Can you work these out from the model? Positions are in its coordinate system, mm. Face numbers are marked on the shaded views. A direction names the side the tool comes from. Give positions to 0.01 mm unless a question says otherwise; leave off trailing zeros. Write each loop counter-clockwise with the first axis right and the second up, starting at its lowest first coordinate (ties: lowest second). Pieces come first, ordered by that corner, then holes.
1. I'm going to push flat-ended pins straight in: pin 1 (2.5 mm diameter, centred on x = 0, z = 10, fed in from -Y); pin 2 (5 mm diameter, centred on x = -50, z = 10, fed in from -Y); pin 3 (2 mm diameter, centred on x = -53.5, y = -2.5, fed in from +Z); pin 4 (4 mm diameter, centred on x = -27.5, z = 8, fed in from -Y). Where does each tip first touch, or does it pass through?
2. Suppose I cut it at A-A (x = -50). Please give me the cut outline in (y, z), and give its area (3 significant figures).
3. If I drill on probe 1 along Z at (x, y) = (-50, -2.4); probe 2 along X at (y, z) = (-1.5, 9.75); probe 3 along Z at (x, y) = (-11, -5.5), over which ranges is the centre line in solid material (lowest first)?
4. On a 3-axis mill with a long thin cutter (end or side, diameter ignored), from which of +Z, -Z, +X, -X, +Y, -Y can I reach the whole of each face in a straight line? I mean the marked faces 5 and 6. Say none if no direction works.
5. Suppose I cut it at B-B (y = -0.5). Please give me the cut outline in (x, z).
6. Suppose I cut it at C-C (z = 10). Please give me the cut outline in (x, y), and give its area (3 significant figures).
7. Suppose I cut it at D-D (x = -41). Please give me the cut outline in (y, z).
8. Thinking about a two-plate mould opening in X: for the marked faces 1, 2, 3 and 4, which applies, pulls with the +X half, pulls with the -X half, needs draft (parallel to the pull), parting line crosses it, or undercut?
```python
from build123d import *

# Parameters (mm, degrees)
F0_R         = 1.5
F1_DEPTH     = 8
F2_T1_DEPTH  = 17.5
F2_T3_DEPTH  = 70
F2_T5_DEPTH  = 7
F2_T7_DEPTH  = 10
F2_T9_DEPTH  = 16
F2_T11_DEPTH = 44
F2_T13_DEPTH = 16
F2_T15_DEPTH = 7
F2_T25_DEPTH = 12
F2_T29_DEPTH = 15
F2_T36_DEPTH = 15
F2_T40_DEPTH = 49
F2_T47_DEPTH = 49
F2_T51_DEPTH = 15
F2_T58_DEPTH = 15
F2_T62_DEPTH = 12


# Not quite as in the source:
# - a fillet or chamfer that OpenCascade refuses, or shapes differently, is made with other operations: its cross-section is extruded or revolved along the edge and cut away or added


with BuildPart() as f1:
    # F0 (on Front) → F1 (new body)
    with BuildSketch(Plane.XZ):
        Polygon((-55, 7.5), (-55, 0), (5, 0), (5, 7.5), (3, 7.5), (3, 12.5), (-3, 12.5), (-3, 7.5), (-47, 7.5), (-47, 12.5), (-53, 12.5), (-53, 7.5), align=None)
        with Locations((-50, 10)):
            Circle(F0_R, mode=Mode.SUBTRACT)
        with Locations((0, 10)):
            Circle(F0_R, mode=Mode.SUBTRACT)
    extrude(amount=F1_DEPTH)

    # F2: fillet of radius 2 on 14 edges, made by hand

    # F2_s2 → F2_t1 (cut)
    with BuildSketch(Plane.XY.offset(-5)):
        with BuildLine():
            ThreePointArc((-55, -6), (-54.4142135624, -7.4142135624), (-53, -8))
            Line((-53, -8), (-55, -8))
            Line((-55, -8), (-55, -6))
        make_face()
        with BuildLine():
            ThreePointArc((5, -6), (4.4142135624, -7.4142135624), (3, -8))
            Line((3, -8), (5, -8))
            Line((5, -8), (5, -6))
        make_face()
    extrude(amount=F2_T1_DEPTH, mode=Mode.SUBTRACT)

    # F2_s4 → F2_t3 (cut)
    with BuildSketch(Plane.YZ.offset(-60)):
        with BuildLine():
            ThreePointArc((-6, 0), (-7.4142135624, 0.5857864376), (-8, 2))
            Line((-8, 2), (-8, 0))
            Line((-8, 0), (-6, 0))
        make_face()
    extrude(amount=F2_T3_DEPTH, mode=Mode.SUBTRACT)

    # F2_s6 → F2_t5 (cut)
    with BuildSketch(Plane.YZ.offset(3)):
        with BuildLine():
            ThreePointArc((-6, 7.5), (-7.4142135624, 6.9142135624), (-8, 5.5))
            Line((-8, 5.5), (-8, 7.5))
            Line((-8, 7.5), (-6, 7.5))
        make_face()
    extrude(amount=F2_T5_DEPTH, mode=Mode.SUBTRACT)

    # F2_s8 → F2_t7 (cut)
    with BuildSketch(Plane.XY.offset(7.5)):
        with BuildLine():
            ThreePointArc((3, -6), (2.4142135624, -7.4142135624), (1, -8))
            Line((1, -8), (3, -8))
            Line((3, -8), (3, -6))
        make_face()
        with BuildLine():
            ThreePointArc((-3, -6), (-2.4142135624, -7.4142135624), (-1, -8))
            Line((-1, -8), (-3, -8))
            Line((-3, -8), (-3, -6))
        make_face()
        with BuildLine():
            ThreePointArc((-47, -6), (-47.5857864376, -7.4142135624), (-49, -8))
            Line((-49, -8), (-47, -8))
            Line((-47, -8), (-47, -6))
        make_face()
        with BuildLine():
            ThreePointArc((-53, -6), (-52.4142135624, -7.4142135624), (-51, -8))
            Line((-51, -8), (-53, -8))
            Line((-53, -8), (-53, -6))
        make_face()
    extrude(amount=F2_T7_DEPTH, mode=Mode.SUBTRACT)

    # F2_s10 → F2_t9 (cut)
    with BuildSketch(Plane.YZ.offset(-8)):
        with BuildLine():
            ThreePointArc((-6, 12.5), (-7.4142135624, 11.9142135624), (-8, 10.5))
            Line((-8, 10.5), (-8, 12.5))
            Line((-8, 12.5), (-6, 12.5))
        make_face()
    extrude(amount=F2_T9_DEPTH, mode=Mode.SUBTRACT)

    # F2_s12 → F2_t11 (cut)
    with BuildSketch(Plane.YZ.offset(-47)):
        with BuildLine():
            ThreePointArc((-6, 7.5), (-7.4142135624, 6.9142135624), (-8, 5.5))
            Line((-8, 5.5), (-8, 7.5))
            Line((-8, 7.5), (-6, 7.5))
        make_face()
    extrude(amount=F2_T11_DEPTH, mode=Mode.SUBTRACT)

    # F2_s14 → F2_t13 (cut)
    with BuildSketch(Plane.YZ.offset(-58)):
        with BuildLine():
            ThreePointArc((-6, 12.5), (-7.4142135624, 11.9142135624), (-8, 10.5))
            Line((-8, 10.5), (-8, 12.5))
            Line((-8, 12.5), (-6, 12.5))
        make_face()
    extrude(amount=F2_T13_DEPTH, mode=Mode.SUBTRACT)

    # F2_s16 → F2_t15 (cut)
    with BuildSketch(Plane.YZ.offset(-60)):
        with BuildLine():
            ThreePointArc((-6, 7.5), (-7.4142135624, 6.9142135624), (-8, 5.5))
            Line((-8, 5.5), (-8, 7.5))
            Line((-8, 7.5), (-6, 7.5))
        make_face()
    extrude(amount=F2_T15_DEPTH, mode=Mode.SUBTRACT)

    # F2_s17 → F2_t18 (revolve, cut)
    with BuildSketch(Plane.XY.offset(10)):
        with BuildLine():
            ThreePointArc((-48.5, -6), (-47.9142135624, -7.4142135624), (-46.5, -8))
            Line((-46.5, -8), (-48.5, -8))
            Line((-48.5, -8), (-48.5, -6))
        make_face()
    revolve(axis=Axis((-50, -8, 10), (0, -1, 0)), mode=Mode.SUBTRACT)

    # F2_s19 → F2_t20 (revolve, cut)
    with BuildSketch(Plane.XY.offset(10)):
        with BuildLine():
            ThreePointArc((1.5, -6), (2.0857864376, -7.4142135624), (3.5, -8))
            Line((3.5, -8), (1.5, -8))
            Line((1.5, -8), (1.5, -6))
        make_face()
    revolve(axis=Axis((0, -8, 10), (0, -1, 0)), mode=Mode.SUBTRACT)


with BuildPart() as f2_tool23:
    # F2_s24 → F2_t25 (new body)
    with BuildSketch(Plane.YZ.offset(10)):
        with BuildLine():
            ThreePointArc((-6, 7.5), (-7.4142135624, 6.9142135624), (-8, 5.5))
            Line((-8, 5.5), (-8, 7.5))
            Line((-8, 7.5), (-6, 7.5))
        make_face()
    extrude(amount=-F2_T25_DEPTH)

    split(bisect_by=Plane.YZ.offset(3), keep=Keep.BOTTOM)


with BuildPart() as f2_tool27:
    # F2_s28 → F2_t29 (new body)
    with BuildSketch(Plane.XY.offset(2.5)):
        with BuildLine():
            ThreePointArc((3, -6), (2.4142135624, -7.4142135624), (1, -8))
            Line((1, -8), (3, -8))
            Line((3, -8), (3, -6))
        make_face()
    extrude(amount=F2_T29_DEPTH)

    split(bisect_by=Plane.XY.offset(7.5), keep=Keep.BOTTOM)


with BuildPart() as f2_tool23_1:
    add(f2_tool23.part)

    # F2_t31: intersect F2_tool27
    add(f2_tool27.part, mode=Mode.INTERSECT)


with BuildPart() as f1_1:
    add(f1.part)

    # F2_t21: cut F2_tool23
    add(f2_tool23_1.part, mode=Mode.SUBTRACT)


with BuildPart() as f2_tool34:
    # F2_s35 → F2_t36 (new body)
    with BuildSketch(Plane.XY.offset(17.5)):
        with BuildLine():
            ThreePointArc((-3, -6), (-2.4142135624, -7.4142135624), (-1, -8))
            Line((-1, -8), (-3, -8))
            Line((-3, -8), (-3, -6))
        make_face()
    extrude(amount=-F2_T36_DEPTH)

    split(bisect_by=Plane.XY.offset(7.5), keep=Keep.BOTTOM)


with BuildPart() as f2_tool38:
    # F2_s39 → F2_t40 (new body)
    with BuildSketch(Plane.YZ.offset(2)):
        with BuildLine():
            ThreePointArc((-6, 7.5), (-7.4142135624, 6.9142135624), (-8, 5.5))
            Line((-8, 5.5), (-8, 7.5))
            Line((-8, 7.5), (-6, 7.5))
        make_face()
    extrude(amount=-F2_T40_DEPTH)

    split(bisect_by=Plane.YZ.offset(-3), keep=Keep.TOP)


with BuildPart() as f2_tool34_1:
    add(f2_tool34.part)

    # F2_t42: intersect F2_tool38
    add(f2_tool38.part, mode=Mode.INTERSECT)


with BuildPart() as f1_2:
    add(f1_1.part)

    # F2_t32: cut F2_tool34
    add(f2_tool34_1.part, mode=Mode.SUBTRACT)


with BuildPart() as f2_tool45:
    # F2_s46 → F2_t47 (new body)
    with BuildSketch(Plane.YZ.offset(-3)):
        with BuildLine():
            ThreePointArc((-6, 7.5), (-7.4142135624, 6.9142135624), (-8, 5.5))
            Line((-8, 5.5), (-8, 7.5))
            Line((-8, 7.5), (-6, 7.5))
        make_face()
    extrude(amount=-F2_T47_DEPTH)

    split(bisect_by=Plane.YZ.offset(-47), keep=Keep.BOTTOM)


with BuildPart() as f2_tool49:
    # F2_s50 → F2_t51 (new body)
    with BuildSketch(Plane.XY.offset(2.5)):
        with BuildLine():
            ThreePointArc((-47, -6), (-47.5857864376, -7.4142135624), (-49, -8))
            Line((-49, -8), (-47, -8))
            Line((-47, -8), (-47, -6))
        make_face()
    extrude(amount=F2_T51_DEPTH)

    split(bisect_by=Plane.XY.offset(7.5), keep=Keep.BOTTOM)


with BuildPart() as f2_tool45_1:
    add(f2_tool45.part)

    # F2_t53: intersect F2_tool49
    add(f2_tool49.part, mode=Mode.INTERSECT)


with BuildPart() as f1_3:
    add(f1_2.part)

    # F2_t43: cut F2_tool45
    add(f2_tool45_1.part, mode=Mode.SUBTRACT)


with BuildPart() as f2_tool56:
    # F2_s57 → F2_t58 (new body)
    with BuildSketch(Plane.XY.offset(17.5)):
        with BuildLine():
            ThreePointArc((-53, -6), (-52.4142135624, -7.4142135624), (-51, -8))
            Line((-51, -8), (-53, -8))
            Line((-53, -8), (-53, -6))
        make_face()
    extrude(amount=-F2_T58_DEPTH)

    split(bisect_by=Plane.XY.offset(7.5), keep=Keep.BOTTOM)


with BuildPart() as f2_tool60:
    # F2_s61 → F2_t62 (new body)
    with BuildSketch(Plane.YZ.offset(-48)):
        with BuildLine():
            ThreePointArc((-6, 7.5), (-7.4142135624, 6.9142135624), (-8, 5.5))
            Line((-8, 5.5), (-8, 7.5))
            Line((-8, 7.5), (-6, 7.5))
        make_face()
    extrude(amount=-F2_T62_DEPTH)

    split(bisect_by=Plane.YZ.offset(-53), keep=Keep.TOP)


with BuildPart() as f2_tool56_1:
    add(f2_tool56.part)

    # F2_t64: intersect F2_tool60
    add(f2_tool60.part, mode=Mode.INTERSECT)


with BuildPart() as f1_4:
    add(f1_3.part)

    # F2_t54: cut F2_tool56
    add(f2_tool56_1.part, mode=Mode.SUBTRACT)


solid = f1_4.part
```
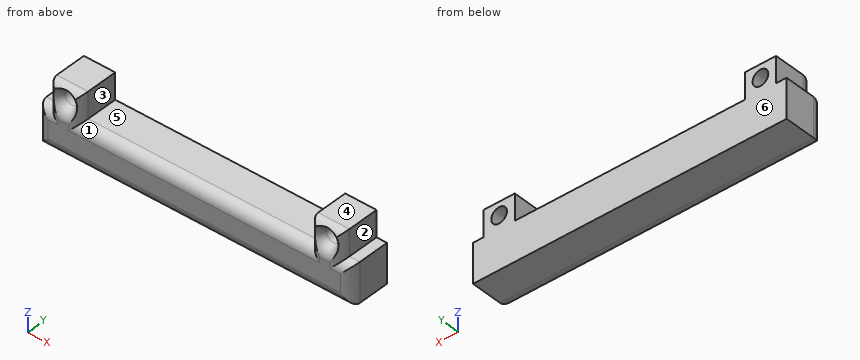
Checks:
1. pin 1: passes through
1. pin 2: stops at y = -7.73
1. pin 3: stops at z = 12.5
1. pin 4: stops at y = -7.94
2. outline: (-8, 2) arc R2 ccw to (-6, 0) - (0, 0) - (0, 8.5) - (-6, 8.5) arc R2 ccw to (-8, 6.5) - close; (-7.32, 12) arc R2 ccw to (-6, 11.5) - (0, 11.5) - (0, 12.5) - (-6, 12.5) arc R2 ccw to start
2. area: 73.2 mm2
3. probe 1: z = 0 to 8.5, 11.5 to 12.5
3. probe 2: x = -53 to -51.48, -48.52 to -47, -3 to -1.48, 1.48 to 3
3. probe 3: z = 0 to 7.5
4. face 5: +Z, +Y, -Y
4. face 6: +Z, -Z, +X, -X, +Y
5. outline: (-55, 0) - (5, 0) - (5, 7.5) - (3, 7.5) - (3, 12.5) - (-3, 12.5) - (-3, 7.5) - (-47, 7.5) - (-47, 12.5) - (-53, 12.5) - (-53, 7.5) - (-55, 7.5) - close; hole circle Ø3 at (-50, 10); hole circle Ø3 at (0, 10)
6. outline: (-53, -6) arc R2 ccw to (-52.25, -7.56) arc R2 ccw to (-51.5, -6) - (-51.5, 0) - (-53, 0) - close; (-48.5, -6) arc R2 ccw to (-47.75, -7.56) arc R2 ccw to (-47, -6) - (-47, 0) - (-48.5, 0) - close; (-3, -6) arc R2 ccw to (-2.25, -7.56) arc R2 ccw to (-1.5, -6) - (-1.5, 0) - (-3, 0) - close; (1.5, -6) arc R2 ccw to (2.25, -7.56) arc R2 ccw to (3, -6) - (3, 0) - (1.5, 0) - close
6. area: 42.5 mm2
7. outline: (-8, 2) arc R2 ccw to (-6, 0) - (0, 0) - (0, 7.5) - (-6, 7.5) arc R2 ccw to (-8, 5.5) - close
8. face 1: undercut
8. face 2: pulls with the +X half
8. face 3: undercut
8. face 4: needs draft
